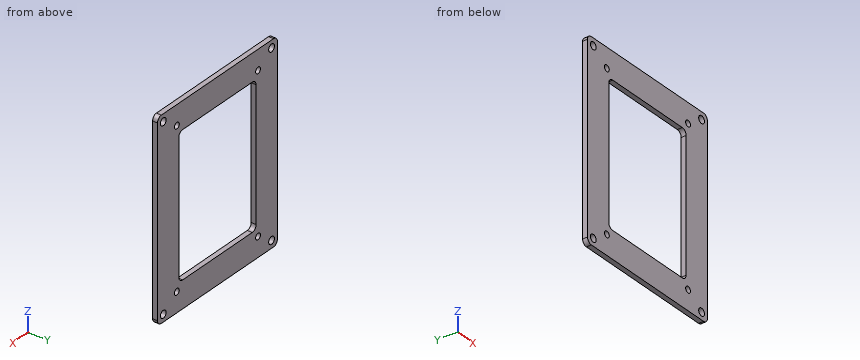
```python
from build123d import *

# Parameters (mm, degrees)
SKETCH_1_W          = 62
SKETCH_1_H          = 79
SKETCH_1_R          = 1.25
EXTRUDE_1_DEPTH     = 2
SKETCH_2_R          = 1.498589197
CUT_EXTRUDE_1_DEPTH = 2
SKETCH_3_W          = 40
SKETCH_3_H          = 57
CUT_EXTRUDE_2_DEPTH = 2
FILLET_1_R          = 2


with BuildPart() as part:
    # 草图1 → 凸台-拉伸1 (new body)
    with BuildSketch(Plane(origin=(0, 0, 0), x_dir=(1, 0, 0), z_dir=(0, 1, 0))):
        Rectangle(SKETCH_1_W, SKETCH_1_H)
        with Locations(Location((-21, 31.5, 0), (0, 0, 270))):
            Circle(SKETCH_1_R, mode=Mode.SUBTRACT)
        with Locations(Location((21, 31.5, 0), (0, 0, 270))):
            Circle(SKETCH_1_R, mode=Mode.SUBTRACT)
        with Locations(Location((-21, -31.5, 0), (0, 0, 270))):
            Circle(SKETCH_1_R, mode=Mode.SUBTRACT)
        with Locations(Location((21, -31.5, 0), (0, 0, 270))):
            Circle(SKETCH_1_R, mode=Mode.SUBTRACT)
    extrude(amount=EXTRUDE_1_DEPTH)

    # 草图2 → 切除-拉伸1 (cut)
    with BuildSketch(Plane(origin=(0, 2, 0), x_dir=(1, 0, 0), z_dir=(0, 1, 0))):
        with Locations(Location((28, 36.5, 0), (0, 0, 270))):
            Circle(SKETCH_2_R)
        with Locations(Location((-28, 36.5, 0), (0, 0, 270))):
            Circle(SKETCH_2_R)
        with Locations(Location((-28, -36.5, 0), (0, 0, 270))):
            Circle(SKETCH_2_R)
        with Locations(Location((28, -36.5, 0), (0, 0, 270))):
            Circle(SKETCH_2_R)
    extrude(amount=-CUT_EXTRUDE_1_DEPTH, mode=Mode.SUBTRACT)

    # 草图3 → 切除-拉伸2 (cut)
    with BuildSketch(Plane(origin=(0, 2, 0), x_dir=(1, 0, 0), z_dir=(0, 1, 0))):
        Rectangle(SKETCH_3_W, SKETCH_3_H)
    extrude(amount=-CUT_EXTRUDE_2_DEPTH, mode=Mode.SUBTRACT)

    # 圆角1
    fillet_1_edges = [part.edges().sort_by_distance(p)[0] for p in [
        (20, 1, -28.5),
        (20, 1, 28.5),
        (-20, 1, 28.5),
        (-20, 1, -28.5),
        (31, 1, 39.5),
        (-31, 1, 39.5),
        (-31, 1, -39.5),
        (31, 1, -39.5),
    ]]
    fillet(fillet_1_edges, radius=FILLET_1_R)


solid = part.part
```
Could you check a few things on this model? Use its own coordinates, in mm. Coordinates: 2 decimals unless noted, no trailing zeros. Write each loop counter-clockwise with the first axis right and the second up, starting at its lowest first coordinate (ties: lowest second). Pieces come first, ordered by that corner, then holes. Notation, with made-up numbers: M 39,-19.5 L 87,-19.5 A24 ccw 87,0.5 Z; hole C -4,68.5 d6. An arc over 180 degrees is marked long. Answer as CSV lines item,"result". Start each with the question number.
1) I want a section at A-A, the plane z = 36.5. Please give me the cut outline in (x, y).
2) I want a section at C-C, the plane z = -5. Please give me the cut outline in (x, y), and give its area (3 significant figures).
3) I want a section at B-B, the plane x = -21. Please give me the cut outline in (y, z), and give its area (3 significant figures).
4) For P1, Ø1.8, axis at x = 28, z = -36.5, coming from the +Y side, with a flat end and sliding along its axis, tell me the tip position at first contact or that it passes through.
5) I want a section at D-D, the plane y = 0.85. Give the number of separate pieces and of enclosed holes in the cut face, and give its area (3 significant figures).
6) Please list where these lines run through material, in increasing order: line 1 (X direction, y = 1.4, z = -36.5); line 2 (X direction, y = 1.55, z = -31.5); line 3 (X direction, y = 0.85, z = 13.5). Write a range as from..to.
Data:
1,outline,"M -31,0 L -29.5,0 L -29.5,2 L -31,2 Z; M -26.5,0 L 26.5,0 L 26.5,2 L -26.5,2 Z; M 29.5,0 L 31,0 L 31,2 L 29.5,2 Z"
2,outline,"M -31,0 L -20,0 L -20,2 L -31,2 Z; M 20,0 L 31,0 L 31,2 L 20,2 Z"
2,area,"44.0 mm^2"
3,outline,"M 0,-39.5 L 2,-39.5 L 2,-32.75 L 0,-32.75 Z; M 0,-30.25 L 2,-30.25 L 2,30.25 L 0,30.25 Z; M 0,32.75 L 2,32.75 L 2,39.5 L 0,39.5 Z"
3,area,"148 mm^2"
4,P1,"passes through"
5,separate pieces,"1"
5,enclosed holes,"9"
5,area,"2,570 mm^2"
6,line 1,"x = -31..-29.5, -26.5..26.5, 29.5..31"
6,line 2,"x = -31..-22.25, -19.75..19.75, 22.25..31"
6,line 3,"x = -31..-20, 20..31"
